from build123d import *

# Parameters (mm, degrees)
BOSS_EXTRUDE1_DEPTH = 10
BOSS_EXTRUDE2_START = -3.5
BOSS_EXTRUDE2_DEPTH = 17
BOSS_EXTRUDE3_START = -5
BOSS_EXTRUDE3_DEPTH = 10
SKETCH6_OUTSIDE_W   = 74.788
SKETCH6_OUTSIDE_H   = 74.788
CUT_EXTRUDE1_DEPTH  = 10
SKETCH5_R           = 10.975
BOSS_EXTRUDE4_DEPTH = 22.28
CHAMFER2_SIZE       = 8.5
CHAMFER2_SIZE_2     = 3


with BuildPart() as part:
    # Sketch1 → Revolve1 (revolve)
    with BuildSketch(Plane(origin=(0, 0, 0), x_dir=(1, 0, 0), z_dir=(0, 1, 0))):
        with BuildLine():
            Line((75.5, 0), (75.5, 10))
            add(Edge.make_bspline(
                [(0, 18.3), (9.740701491, 18.3), (26.990075189, 17.742872667), (54.88230213, 14.080751962), (69.777131961, 10), (75.5, 10)],
                knots=[0, 0, 0, 0, 0.31632777, 0.808812889, 1, 1, 1, 1], degree=3))
            Line((0, 18.3), (0, 0))
            Line((0, 0), (75.5, 0))
        make_face()
    revolve(axis=Axis((0, 0, 0), (1, 0, 0)))

    # Sketch2 → Boss-Extrude1 (add)
    with BuildSketch(Plane(origin=(75.5, 0, 0), x_dir=(0, 0, -1), z_dir=(1, 0, 0))):
        with BuildLine():
            Line((-11.5, 0), (-11.5, -19))
            ThreePointArc((-11.5, -19), (-8.131727984, -27.131727984), (0, -30.5))
            Line((0, -30.5), (19, -30.5))
            ThreePointArc((19, -30.5), (30.5, -19), (19, -7.5))
            Line((19, -7.5), (11.5, -7.5))
            Line((11.5, -7.5), (11.5, 0))
            ThreePointArc((11.5, 0), (0, 11.5), (-11.5, 0))
        make_face()
    extrude(amount=BOSS_EXTRUDE1_DEPTH)

    # Sketch3 → Boss-Extrude2 (add)
    with BuildSketch(Plane.XY.offset(11.5).offset(BOSS_EXTRUDE2_START)):
        Polygon((85.5, -27.9), (98.1, -15.3), (98.1, -3.7), (85.5, 8.9), align=None)
    extrude(amount=-BOSS_EXTRUDE2_DEPTH)

    # Sketch4 → Boss-Extrude3 (add)
    with BuildSketch(Plane(origin=(0, -30.5, 0), x_dir=(-1, 0, 0), z_dir=(0, -1, 0)).offset(BOSS_EXTRUDE3_START)):
        Polygon((-75.5, -6.49101914), (-61.854263107, 7.154717753), (-61.854263107, 15.856079818), (-75.5, 29.50181671), align=None)
    extrude(amount=-BOSS_EXTRUDE3_DEPTH)

    # Sketch6 outside → Cut-Extrude1 (cut)
    with BuildSketch(Plane(origin=(85.5, 0, 0), x_dir=(0, 0, -1), z_dir=(1, 0, 0))):
        with Locations((6.1, -6.1)):
            Rectangle(SKETCH6_OUTSIDE_W, SKETCH6_OUTSIDE_H)
        with BuildLine():
            Line((8.423507913, 0.476492087), (8.423507913, -19.476492087))
            ThreePointArc((8.423507913, -19.476492087), (0, -27.9), (-8.423507913, -19.476492087))
            Line((-8.423507913, -19.476492087), (-8.423507913, 0.476492087))
            ThreePointArc((-8.423507913, 0.476492087), (0, 8.9), (8.423507913, 0.476492087))
        make_face(mode=Mode.SUBTRACT)
    extrude(amount=CUT_EXTRUDE1_DEPTH, mode=Mode.SUBTRACT)

    # Sketch5 → Boss-Extrude4 (add)
    with BuildSketch(Plane(origin=(85.5, 0, 0), x_dir=(0, 0, -1), z_dir=(1, 0, 0))):
        with Locations(Location((19, -19, 0), (0, 0, 191.531863493))):
            Circle(SKETCH5_R)
    extrude(amount=BOSS_EXTRUDE4_DEPTH)

    # Chamfer2
    # the kernel refuses this chamfer: 8.5, 3 mm, written as the material it takes off along each edge
    with BuildSketch(Plane(origin=(98.1, -37.353356339, 8), x_dir=(-0.9999177197745295, 0, 0.012827847867252683), z_dir=(0, 1, 0))) as chamfer2_piece_1:
        Polygon((CHAMFER2_SIZE * 0.999917719775, -CHAMFER2_SIZE * 0.0128278478673), (-CHAMFER2_SIZE_2 * 0.0128278478673, -CHAMFER2_SIZE_2 * 0.999917719775), (0, 0), align=None)
    extrude(amount=55.706712677, mode=Mode.SUBTRACT)


solid = part.part
Input: part model. Units: mm. Frame: model coordinates. A direction names the side the tool comes from. Give positions to 0.01 mm unless a question says otherwise; leave off trailing zeros. Use one line per item in the form item = value.
1) Line query: probe 1 along X at (y, z) = (-24, -8); probe 2 along Y at (x, z) = (73, -26.5); probe 3 along Y at (x, z) = (77, 0.5). Output: solid intervals per line, ascending.
Response values:
probe_1 = 61.85 to 85.5
probe_2 = -25.5 to -15.5
probe_3 = -30.49 to 11.49
2) First-contact query: pin 1 Ø4.5 at (x, y) = (88.5, -12) entering from +Z; pin 2 Ø2 at (x, y) = (80, -3) entering from -Z; pin 3 Ø3 at (x, y) = (88.5, -12) entering from -Z; pin 4 Ø15 at (x, z) = (71.5, -2.5) entering from -Y. Flat tips, straight axial feed; report the tip coordinate or a pass-through.
Response values:
pin_1 = 8
pin_2 = -11.5
pin_3 = -28.5
pin_4 = -30.5
3) Mould query, pull axis X, two halves, no side actions, for faces 6 (the flat face through (70, -15.5, -12)), 7 (the flat face through (69, -21, -23)), 8 (the flat face through (88, -9, 8)). Classes: pulls with the +X half, pulls with the -X half, needs draft (parallel to the pull), parting line crosses it, or undercut.
Response values:
face_6 = undercut
face_7 = pulls with the -X half
face_8 = needs draft
4) Reachability of faces 1 (the flat face through (70, -25.5, -12)), 2 (the cylindrical face through (87.403, -24.741, 6.576)), 3 (the flat face through (75.5, -14, -5)), 4 (the cylindrical face through (87.4, 5.62, 6.67)), 5 (the flat face through (68.77, -20.57, -0.24)) from +Z, -Z, +X, -X, +Y, -Y: full face, straight path, thin tool, end or side. Return the list, or none.
Response values:
face_1 = +Z, -Z, -X, -Y
face_2 = +Z, +X, -Y
face_3 = none
face_4 = +Z, +X, +Y
face_5 = +Z, -Y
